The model under review builds one solid part; all positions refer to its coordinate system, in mm. A direction names the side the tool comes from. Coordinates: 2 decimals unless noted, no trailing zeros. Write each loop counter-clockwise with the first axis right and the second up, starting at its lowest first coordinate (ties: lowest second). Pieces come first, ordered by that corner, then holes. Notation, with made-up numbers: M -28,8 L -15,8 A18 cw -15,12 Z; hole C 86.25,69.5 d2. An arc over 180 degrees is marked long. Answer as a JSON object with one key per item and string values.
```python
from build123d import *

# Parameters (mm, degrees)
F1_DEPTH = 279.4
F3_DEPTH = 25.401
F5_D     = 19.05


# Not quite as in the source:
# - a feature names something its author has since deleted; it is built from what else it names


with BuildPart() as f1:
    # F0 (on Front) → F1 (new body)
    with BuildSketch(Plane.XZ):
        Polygon((25.4, -12.7), (25.4, 12.7), (-25.4, 12.7), (-25.4, -12.7), (-22.225, -12.7), (-22.225, 9.525), (22.225, 9.525), (22.225, -12.7), align=None)
    extrude(amount=F1_DEPTH)

    # F2 (on face) → F3 (cut, through all)
    with BuildSketch(Plane.XY.offset(12.7)):
        with BuildLine():
            Line((0, -40.4343813046), (9.525, -40.4343813046))
            ThreePointArc((9.525, -40.4343813046), (6.7351920908, -33.6991892138), (0, -30.9093813046))
            Line((0, -30.9093813046), (0, -40.4343813046))
        make_face()
        with BuildLine():
            ThreePointArc((0, -30.9093813046), (-6.7351920908, -33.6991892138), (-9.525, -40.4343813046))
            Line((-9.525, -40.4343813046), (0, -40.4343813046))
            Line((0, -40.4343813046), (0, -30.9093813046))
        make_face()
        with BuildLine():
            Line((0, -40.4343813046), (-9.525, -40.4343813046))
            ThreePointArc((-9.525, -40.4343813046), (-6.7351920908, -47.1695733954), (0, -49.9593813046))
            Line((0, -49.9593813046), (0, -40.4343813046))
        make_face()
        with BuildLine():
            Line((0, -103.9343813046), (9.525, -103.9343813046))
            ThreePointArc((9.525, -103.9343813046), (6.7351920908, -97.1991892138), (0, -94.4093813046))
            Line((0, -94.4093813046), (0, -103.9343813046))
        make_face()
        with BuildLine():
            ThreePointArc((0, -94.4093813046), (-6.7351920908, -97.1991892138), (-9.525, -103.9343813046))
            Line((-9.525, -103.9343813046), (0, -103.9343813046))
            Line((0, -103.9343813046), (0, -94.4093813046))
        make_face()
        with BuildLine():
            ThreePointArc((0, -113.4593813046), (6.7351920908, -110.6695733954), (9.525, -103.9343813046))
            Line((9.525, -103.9343813046), (0, -103.9343813046))
            Line((0, -103.9343813046), (0, -113.4593813046))
        make_face()
        with BuildLine():
            Line((0, -103.9343813046), (-9.525, -103.9343813046))
            ThreePointArc((-9.525, -103.9343813046), (-6.7351920908, -110.6695733954), (0, -113.4593813046))
            Line((0, -113.4593813046), (0, -103.9343813046))
        make_face()
        with BuildLine():
            Line((0, -167.4343813046), (9.525, -167.4343813046))
            ThreePointArc((9.525, -167.4343813046), (6.7351920908, -160.6991892138), (0, -157.9093813046))
            Line((0, -157.9093813046), (0, -167.4343813046))
        make_face()
        with BuildLine():
            ThreePointArc((0, -157.9093813046), (-6.7351920908, -160.6991892138), (-9.525, -167.4343813046))
            Line((-9.525, -167.4343813046), (0, -167.4343813046))
            Line((0, -167.4343813046), (0, -157.9093813046))
        make_face()
        with BuildLine():
            Line((0, -167.4343813046), (0, -176.9593813046))
            ThreePointArc((0, -176.9593813046), (6.7351920908, -174.1695733954), (9.525, -167.4343813046))
            Line((9.525, -167.4343813046), (0, -167.4343813046))
        make_face()
        with BuildLine():
            ThreePointArc((-9.525, -167.4343813046), (-6.7351920908, -174.1695733954), (0, -176.9593813046))
            Line((0, -176.9593813046), (0, -167.4343813046))
            Line((0, -167.4343813046), (-9.525, -167.4343813046))
        make_face()
        with BuildLine():
            Line((0, -220.9396968842), (0, -230.4646968842))
            Line((0, -230.4646968842), (9.525, -230.4646968842))
            ThreePointArc((9.525, -230.4646968842), (6.7351920908, -223.7295047934), (0, -220.9396968842))
        make_face()
        with BuildLine():
            Line((-9.525, -230.4646968842), (0, -230.4646968842))
            Line((0, -230.4646968842), (0, -220.9396968842))
            ThreePointArc((0, -220.9396968842), (-6.7351920908, -223.7295047934), (-9.525, -230.4646968842))
        make_face()
        with BuildLine():
            ThreePointArc((0, -49.9593813046), (6.7351920908, -47.1695733954), (9.525, -40.4343813046))
            Line((9.525, -40.4343813046), (0, -40.4343813046))
            Line((0, -40.4343813046), (0, -49.9593813046))
        make_face()
    extrude(amount=-F3_DEPTH, mode=Mode.SUBTRACT)

    # F5 (through all)
    with Locations(Plane.XY.offset(12.7)):
        with Locations((0, -230.4646968842)):
            Hole(F5_D / 2)


solid = f1.part
```
(1) Add section A-A on z = -2.5. Give the boundary of the cut face in (x, y) (3 decimals), and give its area (3 significant figures).
Results list:
{"outline": "M -25.4,-279.4 L -22.225,-279.4 L -22.225,0 L -25.4,0 Z; M 22.225,-279.4 L 25.4,-279.4 L 25.4,0 L 22.225,0 Z", "area": "1,770 mm²"}
(2) For pin 1 Ø22 at (x, y) = (-4, -82.5) entering from -Z (3 decimals), flat-tipped, find the tip position at first contact; note if it passes through.
Results list:
{"pin 1": "z = 9.525"}
(3) For faces 1 (the face through (25.4, -138, 0)), 2 (the face through (22.225, -138, -1)), list the 3-axis set-ups (+Z, -Z, +X, -X, +Y, -Y) from which the entire face can be reached by the end or side of a thin tool; tool diameter is ignored.
Results list:
{"face 1": "+Z, -Z, +X, +Y, -Y", "face 2": "-Z, +Y, -Y"}
(4) Draft analysis for pull direction Y (two halves, no side actions). For faces 3 (the face through (0, -279.4, 10)), 4 (the face through (0, -138, 12.7)), 5 (the face through (-2.065, -239.763, 11.135)), state which applies: released by +Y, released by -Y, zero draft, split by the parting line, or undercut.
Results list:
{"face 3": "released by -Y", "face 4": "zero draft", "face 5": "undercut"}
(5) Add section B-B on y = -217. Give the boundary of the cut face in (x, z) (3 decimals), and give its area (3 significant figures).
Results list:
{"outline": "M -25.4,-12.7 L -22.225,-12.7 L -22.225,9.525 L 22.225,9.525 L 22.225,-12.7 L 25.4,-12.7 L 25.4,12.7 L -25.4,12.7 Z", "area": "302 mm²"}
(6) Wall thickness on line 1 along X through (y, z) = (-208, -7.25) (3 decimals); line 2 along Z through (x, y) = (5, -250) (3 decimals): over which ranges is each line inside the solid? List them lowest first. Write a range as from..to.
Results list:
{"line 1": "-25.4..-22.225, 22.225..25.4", "line 2": "9.525..12.7"}
(7) Add section C-C on x = 12. Give the boundary of the cut face in (y, z) (3 decimals), and give its area (3 significant figures).
Results list:
{"outline": "M -279.4,9.525 L 0,9.525 L 0,12.7 L -279.4,12.7 Z", "area": "887 mm²"}
